```python
from build123d import *

# Parameters (mm, degrees)
SKETCH_1_R          = 2
SKETCH_1_R_2        = 1
EXTRUDE_1_DEPTH     = 1.6
SKETCH_2_R          = 2.5
EXTRUDE_2_DEPTH     = 5
SKETCH_3_R          = 2
CUT_EXTRUDE_1_DEPTH = 3.4
SKETCH_4_R          = 1
CUT_EXTRUDE_2_DEPTH = 3.4


with BuildPart() as part:
    # 草图1 → 凸台-拉伸1 (new body)
    with BuildSketch(Plane.XY):
        Circle(SKETCH_1_R)
        Circle(SKETCH_1_R_2, mode=Mode.SUBTRACT)
    extrude(amount=EXTRUDE_1_DEPTH)

    # 草图2 → 凸台-拉伸2 (add)
    with BuildSketch(Plane.XY):
        Circle(SKETCH_2_R)
    extrude(amount=EXTRUDE_2_DEPTH)

    # 草图3 → 切除-拉伸1 (cut)
    with BuildSketch(Plane.XY.offset(5)):
        Circle(SKETCH_3_R)
    extrude(amount=-CUT_EXTRUDE_1_DEPTH, mode=Mode.SUBTRACT)

    # 草图4 → 切除-拉伸2 (cut)
    with BuildSketch(Plane.XY.offset(1.6)):
        Circle(SKETCH_4_R)
    extrude(amount=-CUT_EXTRUDE_2_DEPTH, mode=Mode.SUBTRACT)


solid = part.part
```
Verification items for the finished model (mm, model axes). A direction names the side the tool comes from. Give positions to 0.01 mm unless a question says otherwise; leave off trailing zeros. Order: outer loops, then holes, each group sorted by start corner. A loop starts at its lowest first (then second) coordinate and runs counter-clockwise, first axis right, second up. Notation, with made-up numbers: (25, 68) -> (44, 68) arc R23 cw to (44, 95) -> close; hole circle Ø2 at (-8.75, -8). An arc over 180 degrees is marked (long way). One line per item, written item: value.
(1) Sectioned sample at D-D on y = 1.2. Record the cut outline in (x, z), then the cut area to 3 significant figures.
Final values:
outline: (-2.19, 0) -> (2.19, 0) -> (2.19, 5) -> (1.6, 5) -> (1.6, 1.6) -> (-1.6, 1.6) -> (-1.6, 5) -> (-2.19, 5) -> close
area: 11.1 mm^2
(2) Draft check along X on faces 1 (the face through (1, -1, 0)), 2 (the face through (-0.54, -2.44, 2.46)), 3 (the face through (0, -2, 3)). Enter one of: pulls with the +X half, pulls with the -X half, needs draft (parallel to the pull), parting line crosses it, or undercut.
Final values:
face 1: needs draft
face 2: parting line crosses it
face 3: undercut
(3) Tool access check on faces 4 (the face through (-1, 2, 5)), 5 (the face through (1, -1, 1.6)). Record the directions out of +Z, -Z, +X, -X, +Y, -Y that give a thin tool (end or side, any length) a straight path to the whole face; none if there is none.
Final values:
face 4: +Z, +X, -X, +Y, -Y
face 5: +Z
(4) Gauge pin test, flat ends, axial feed: pin 1 (2 mm diameter, centred on x = 1.5, z = 2, fed in from -Y); pin 2 (2 mm diameter, centred on x = -0.5, y = -0.5, fed in from +Z); pin 3 (1.5 mm diameter, centred on x = 1, z = 3.5, fed in from -Y). Record the tip position at first contact, or that the pin passes through.
Final values:
pin 1: y = -2.45
pin 2: z = 1.6
pin 3: y = -2.49
(5) Sectioned sample at C-C on z = 3.7. Record the cut outline in (x, y), then the cut area to 3 significant figures.
Final values:
outline: circle Ø5 at (0, 0); hole circle Ø4 at (0, 0)
area: 7.07 mm^2
(6) Sectioned sample at A-A on y = 0. Record the cut outline in (x, z).
Final values:
outline: (-2.5, 0) -> (-1, 0) -> (-1, 1.6) -> (-2, 1.6) -> (-2, 5) -> (-2.5, 5) -> close; (1, 0) -> (2.5, 0) -> (2.5, 5) -> (2, 5) -> (2, 1.6) -> (1, 1.6) -> close
(7) Scan lines: line 1 along Z through (x, y) = (-0.2, -1.6); line 2 along X through (y, z) = (0.25, 2); line 3 along Y through (x, z) = (0.85, 2). Record each from-to range of solid material in increasing order. Write a range as [from, to].
Final values:
line 1: [0, 1.6]
line 2: [-2.49, -1.98], [1.98, 2.49]
line 3: [-2.35, -1.81], [1.81, 2.35]
